from build123d import *

# Parameters (mm, degrees)
SKETCH_1_R      = 1.1
EXTRUDE_1_DEPTH = 0.6


with BuildPart() as part:
    # 草图1 → 凸台-拉伸1 (new body)
    with BuildSketch(Plane.XY):
        with BuildLine():
            Line((-26.5, -26.5), (-20.5, -26.5))
            Line((-20.5, -26.5), (-20.5, -18.5))
            Line((-20.5, -18.5), (20.5, -18.5))
            Line((20.5, -18.5), (20.5, -26.5))
            Line((20.5, -26.5), (26.5, -26.5))
            ThreePointArc((26.5, -26.5), (28.267766953, -25.767766953), (29, -24))
            Line((29, -24), (29, 24))
            ThreePointArc((29, 24), (28.267766953, 25.767766953), (26.5, 26.5))
            Line((26.5, 26.5), (-26.5, 26.5))
            ThreePointArc((-26.5, 26.5), (-28.267766953, 25.767766953), (-29, 24))
            Line((-29, 24), (-29, -24))
            ThreePointArc((-29, -24), (-28.267766953, -25.767766953), (-26.5, -26.5))
        make_face()
        with Locations((-26.9, 24.4)):
            Circle(SKETCH_1_R, mode=Mode.SUBTRACT)
        with Locations(Location((-26.9, -24.4, 0), (0, 0, 180))):
            Circle(SKETCH_1_R, mode=Mode.SUBTRACT)
        with Locations((26.9, -24.4)):
            Circle(SKETCH_1_R, mode=Mode.SUBTRACT)
        with Locations(Location((26.9, 24.4, 0), (0, 0, 180))):
            Circle(SKETCH_1_R, mode=Mode.SUBTRACT)
    extrude(amount=EXTRUDE_1_DEPTH)


solid = part.part
The listing builds one solid part. Answer for the finished solid, in the listing's coordinates (mm). Round coordinates to 2 decimals unless told otherwise and drop trailing zeros. Write each loop counter-clockwise with the first axis right and the second up, starting at its lowest first coordinate (ties: lowest second). Pieces come first, ordered by that corner, then holes. Notation, with made-up numbers: M 30,54 L 69,54 A7 ccw 69,58 Z; hole C 44.5,58.5 d4. An arc over 180 degrees is marked long. Write each question's results on one line, items separated by ' | '. Start each with the question number.
(1) Determine the mould class of faces 1 (the cylindrical face through (28.287, 25.748, 0.296)), 2 (the cylindrical face through (26.76, -23.31, 0.3)), 3 (the cylindrical face through (-28.287, -25.748, 0.296)), 4 (the cylindrical face through (-27.49, -25.33, 0.3)) for opening direction X: +X half, -X half, draft (parallel to the pull), parting line (faces both ways), or undercut.
(2) Find the intervals of material crossed by line 1 (Y direction, x = -26.9, z = 0.35); line 2 (Y direction, x = 13, z = 0.55), in increasing order.
(3) Each of these flat-tipped pins is pushed along its axis until it touches: P1, Ø3, axis at x = -26.9, y = 24.4, coming from the -Z side; P2, Ø2, axis at x = 26.9, y = 24.4, coming from the -Z side. Where does it stop, or does it pass through?
(4) The part is cut by section B-B, the plane x = 1. Write down the section's boundary in (y, z), and give its area (3 significant figures).
(5) The part is cut by section A-A, the plane z = 0.15. Write down the section's boundary in (x, y).
Worked answers:
1) face 1: +X half | face 2: undercut | face 3: -X half | face 4: undercut
2) line 1: y = -26.47 to -25.5, -23.3 to 23.3, 25.5 to 26.47 | line 2: y = -18.5 to 26.5
3) P1: stops at z = 0 | P2: passes through
4) outline: M -18.5,0 L 26.5,0 L 26.5,0.6 L -18.5,0.6 Z | area: 27.0 mm²
5) outline: M -29,-24 A2.5 ccw -26.5,-26.5 L -20.5,-26.5 L -20.5,-18.5 L 20.5,-18.5 L 20.5,-26.5 L 26.5,-26.5 A2.5 ccw 29,-24 L 29,24 A2.5 ccw 26.5,26.5 L -26.5,26.5 A2.5 ccw -29,24 Z; hole C -26.9,-24.4 d2.2; hole C -26.9,24.4 d2.2; hole C 26.9,-24.4 d2.2; hole C 26.9,24.4 d2.2
